The model under review builds one solid part; all positions refer to its coordinate system, in mm. Coordinates: 2 decimals unless noted, no trailing zeros. Write each loop counter-clockwise with the first axis right and the second up, starting at its lowest first coordinate (ties: lowest second). Pieces come first, ordered by that corner, then holes. Notation, with made-up numbers: (44.5, -7) - (53.5, -7) arc R30 cw to (53.5, 28) - close; hole circle Ø1 at (-40, 40.25). An arc over 180 degrees is marked (long way). Return JSON: item names as keys, results as strings. Group by question number.
(1) We need section A-A on x = 0. State the section outline as (y, z) points, then the cut area to 3 significant figures.
(2) To check wall thickness, follow L1, parallel to Y at x = 0, z = 28; L2, parallel to Y at x = 4.75, z = 82; L3, parallel to X at y = 4, z = 10. State the ranges of each line that lie inside material, in increasing order. Write a range as from..to.
(3) We need section C-C on x = -4.5. State the section outline as (y, z) points, then the cut area to 3 significant figures.
(4) For pin 1 Ø0.6 at (y, z) = (-9.5, 59) entering from +X; pin 2 Ø12 at (x, y) = (-2, 1) entering from -Z; pin 3 Ø0.6 at (y, z) = (-3, 50) entering from +X; pin 4 Ø1.6 at (y, z) = (9, 26.5) entering from -X, all flat-tipped, find the tip position at first contact; note any pin that passes through.
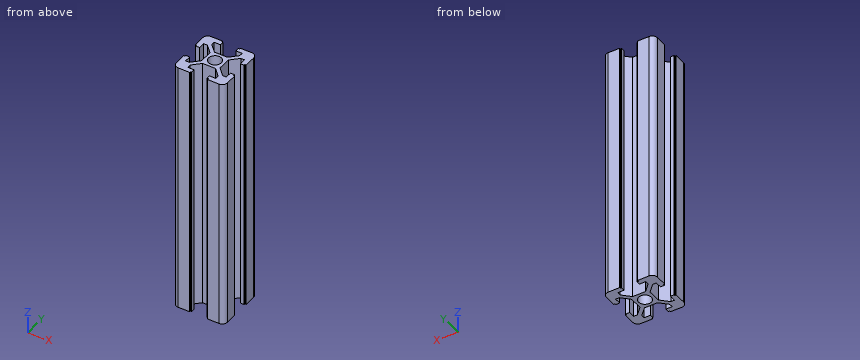
```python
from build123d import *

# Parameters (mm, degrees)
SKETCH1_R           = 2.5
BOSS_EXTRUDE1_DEPTH = 100


with BuildPart() as part:
    # Sketch1 → Boss-Extrude1 (new body)
    with BuildSketch(Plane.XY):
        with BuildLine():
            Line((8, -3), (8, -5.5))
            Line((8, -5.5), (6.560660172, -5.5))
            Line((6.560660172, -5.5), (3.6, -2.539339828))
            Line((3.6, -2.539339828), (3.6, 2.539339828))
            Line((3.6, 2.539339828), (6.560660172, 5.5))
            Line((6.560660172, 5.5), (8, 5.5))
            Line((8, 5.5), (8, 3))
            Line((8, 3), (9.5, 3))
            Line((9.5, 3), (9.5, 3.5))
            Line((9.5, 3.5), (10, 3.5))
            Line((10, 3.5), (10, 8))
            ThreePointArc((10, 8), (9.414213562, 9.414213562), (8, 10))
            Line((8, 10), (3.5, 10))
            Line((3.5, 10), (3.5, 9.5))
            Line((3.5, 9.5), (3, 9.5))
            Line((3, 9.5), (3, 8))
            Line((3, 8), (5.5, 8))
            Line((5.5, 8), (5.5, 6.560660172))
            Line((5.5, 6.560660172), (2.539339828, 3.6))
            Line((2.539339828, 3.6), (-2.539339828, 3.6))
            Line((-2.539339828, 3.6), (-5.5, 6.560660172))
            Line((-5.5, 6.560660172), (-5.5, 8))
            Line((-5.5, 8), (-3, 8))
            Line((-3, 8), (-3, 9.5))
            Line((-3, 9.5), (-3.5, 9.5))
            Line((-3.5, 9.5), (-3.5, 10))
            Line((-3.5, 10), (-8, 10))
            ThreePointArc((-8, 10), (-9.414213562, 9.414213562), (-10, 8))
            Line((-10, 8), (-10, 3.5))
            Line((-10, 3.5), (-9.5, 3.5))
            Line((-9.5, 3.5), (-9.5, 3))
            Line((-9.5, 3), (-8, 3))
            Line((-8, 3), (-8, 5.5))
            Line((-8, 5.5), (-6.560660172, 5.5))
            Line((-6.560660172, 5.5), (-3.6, 2.539339828))
            Line((-3.6, 2.539339828), (-3.6, -2.539339828))
            Line((-3.6, -2.539339828), (-6.560660172, -5.5))
            Line((-6.560660172, -5.5), (-8, -5.5))
            Line((-8, -5.5), (-8, -3))
            Line((-8, -3), (-9.5, -3))
            Line((-9.5, -3), (-9.5, -3.5))
            Line((-9.5, -3.5), (-10, -3.5))
            Line((-10, -3.5), (-10, -8))
            ThreePointArc((-10, -8), (-9.414213562, -9.414213562), (-8, -10))
            Line((-8, -10), (-3.5, -10))
            Line((-3.5, -10), (-3.5, -9.5))
            Line((-3.5, -9.5), (-3, -9.5))
            Line((-3, -9.5), (-3, -8))
            Line((-3, -8), (-5.5, -8))
            Line((-5.5, -8), (-5.5, -6.560660172))
            Line((-5.5, -6.560660172), (-2.539339828, -3.6))
            Line((-2.539339828, -3.6), (2.539339828, -3.6))
            Line((2.539339828, -3.6), (5.5, -6.560660172))
            Line((5.5, -6.560660172), (5.5, -8))
            Line((5.5, -8), (3, -8))
            Line((3, -8), (3, -9.5))
            Line((3, -9.5), (3.5, -9.5))
            Line((3.5, -9.5), (3.5, -10))
            Line((3.5, -10), (8, -10))
            ThreePointArc((8, -10), (9.414213562, -9.414213562), (10, -8))
            Line((10, -8), (10, -3.5))
            Line((10, -3.5), (9.5, -3.5))
            Line((9.5, -3.5), (9.5, -3))
            Line((9.5, -3), (8, -3))
        make_face()
        Circle(SKETCH1_R, mode=Mode.SUBTRACT)
    extrude(amount=BOSS_EXTRUDE1_DEPTH)


solid = part.part
```
Ans:
{
 "1": {"outline": "(-3.6, 0) - (-2.5, 0) - (-2.5, 100) - (-3.6, 100) - close; (2.5, 0) - (3.6, 0) - (3.6, 100) - (2.5, 100) - close", "area": "220 mm²"},
 "2": {"L1": "-3.6..-2.5, 2.5..3.6", "L2": "-10..-8, -5.81..-3.69, 3.69..5.81, 8..10", "L3": "-10..-8, -5.06..-2.94, 2.94..5.06, 8..10"},
 "3": {"outline": "(-10, 0) - (-8, 0) - (-8, 100) - (-10, 100) - close; (-5.56, 0) - (-3.44, 0) - (-3.44, 100) - (-5.56, 100) - close; (3.44, 0) - (5.56, 0) - (5.56, 100) - (3.44, 100) - close; (8, 0) - (10, 0) - (10, 100) - (8, 100) - close", "area": "824 mm²"},
 "4": {"pin 1": "x = 9.6", "pin 2": "z = 0", "pin 3": "x = 9.5", "pin 4": "x = -9.99"}
}
